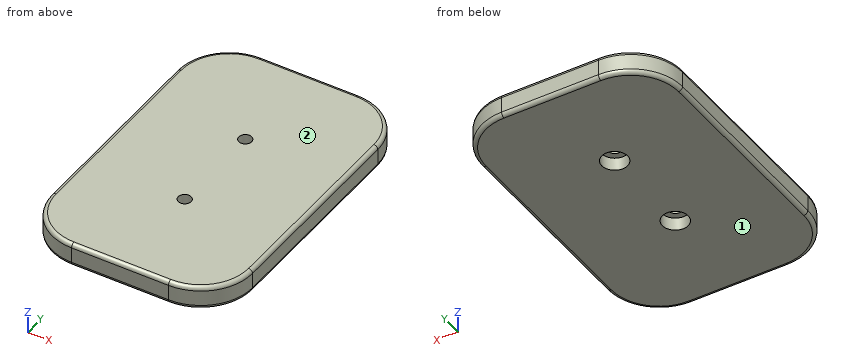
from build123d import *

# Parameters (mm, degrees)
F0_R     = 5
F1_DEPTH = 18
F2_R     = 10
F3_DEPTH = 10
F4_R     = 3


with BuildPart() as f1:
    # F0 (on Top) → F1 (new body)
    with BuildSketch(Plane.XY):
        with BuildLine():
            ThreePointArc((-72.732671, -78.195973), (-61.016942, -106.480244), (-32.732671, -118.195973))
            Line((-32.732671, -118.195973), (42.267329, -118.195973))
            ThreePointArc((42.267329, -118.195973), (70.5516, -106.480244), (82.267329, -78.195973))
            Line((82.267329, -78.195973), (82.267329, 76.804027))
            ThreePointArc((82.267329, 76.804027), (70.5516, 105.088298), (42.267329, 116.804027))
            Line((42.267329, 116.804027), (-32.732671, 116.804027))
            ThreePointArc((-32.732671, 116.804027), (-61.016942, 105.088298), (-72.732671, 76.804027))
            Line((-72.732671, 76.804027), (-72.732671, -78.195973))
        make_face()
        with Locations((4.767329, -38.195973)):
            Circle(F0_R, mode=Mode.SUBTRACT)
        with Locations((4.767329, 36.804027)):
            Circle(F0_R, mode=Mode.SUBTRACT)
    extrude(amount=F1_DEPTH)

    # F2 (on face) → F3 (cut)
    with BuildSketch(Plane(origin=(0, 0, 0), x_dir=(1, 0, 0), z_dir=(0, 0, -1))):
        with Locations((4.767329, 38.195973)):
            Circle(F2_R)
        with Locations((4.767329, -36.804027)):
            Circle(F2_R)
    extrude(amount=-F3_DEPTH, mode=Mode.SUBTRACT)

    # F4
    f4_edges = [f1.edges().sort_by_distance(p)[0] for p in [
        (82.267329, -0.695973, 18),
        (82.267329, -0.695973, 0),
    ]]
    fillet(f4_edges, radius=F4_R)


solid = f1.part
Geometry: final body of the model. Coordinates: model frame, mm. Face numbers are marked on the shaded views. Give positions to 0.01 mm unless a question says otherwise; leave off trailing zeros. Loops run counter-clockwise (first coordinate to the right, second up) from the corner with the lowest first, then second, coordinate; pieces in that order, holes last. Notation, with made-up numbers: (20, 31.5) - (66, 31.5) arc R30 cw to (66, 60.5) - close; hole circle Ø10 at (16.25, 37.5). An arc over 180 degrees is marked (long way). One line per question, with ' | ' between items. Start each with the question number.
(1) Contact query for flat-ended pins moving along their axis: pin 1 (11.5 mm diameter, centred on x = 4.77, y = 36.8, fed in from -Z); pin 2 (10 mm diameter, centred on x = 49, z = 16, fed in from -Y). Output: stop coordinate, or through.
(2) Pull-direction query (Z, two-part tool) for the marked faces 1 and 2; classes: released by +Z, released by -Z, zero draft, split by the parting line, or undercut.
(3) Section query A-A on x = 2.5. Return loops of the section in (y, z).
(4) Ray query, line 1 (Y direction, x = 5, z = 15.5); line 2 (Y direction, x = 7.5, z = 9); line 3 (Y direction, x = -32, z = 15.5). Return the intervals inside material, ascending. Write a range as from..to.
The answers:
1) pin 1: z = 10 | pin 2: y = -118.15
2) face 1: released by -Z | face 2: released by +Z
3) outline: (-118.2, 3) arc R3 ccw to (-115.2, 0) - (-47.94, 0) - (-47.94, 10) - (-42.65, 10) - (-42.65, 18) - (-115.2, 18) arc R3 ccw to (-118.2, 15) - close; (-33.74, 10) - (-28.46, 10) - (-28.46, 0) - (27.06, 0) - (27.06, 10) - (32.35, 10) - (32.35, 18) - (-33.74, 18) - close; (41.26, 10) - (46.54, 10) - (46.54, 0) - (113.8, 0) arc R3 ccw to (116.8, 3) - (116.8, 15) arc R3 ccw to (113.8, 18) - (41.26, 18) - close
4) line 1: -118.15..-43.19, -33.2..31.81, 41.8..116.76 | line 2: -118.2..-47.82, -28.58..27.18, 46.42..116.8 | line 3: -118.15..116.76
